```python
from build123d import *

# Parameters (mm, degrees)
F2_R    = 1
F3_SIZE = 1
F4_SIZE = 0.5


with BuildPart() as f1:
    # F0 (on Front) → F1 (revolve)
    with BuildSketch(Plane.XZ):
        Polygon((0, 7.5), (-10.669873, 7.5), (-15, 0), (0, 0), (0, 2), (15, 2), (15, 4), (0, 4), align=None)
    revolve(axis=Axis((-7.5, 0, 0), (1, 0, 0)))

    # F2
    f2_edges = [f1.edges().sort_by_distance(p)[0] for p in [
        (-10.669873, 0, -7.5),
    ]]
    fillet(f2_edges, radius=F2_R)

    # F3
    f3_edges = [f1.edges().sort_by_distance(p)[0] for p in [
        (0, 0, -7.5),
    ]]
    chamfer(f3_edges, length=F3_SIZE)

    # F4
    f4_edges = [f1.edges().sort_by_distance(p)[0] for p in [
        (15, 0, -4),
    ]]
    chamfer(f4_edges, length=F4_SIZE)


solid = f1.part
```
Check sheet for the modelled part. Datum: model origin and axes. Units: mm. A direction names the side the tool comes from. Coordinates: 2 decimals unless noted, no trailing zeros. Order: outer loops, then holes, each group sorted by start corner. A loop starts at its lowest first (then second) coordinate and runs counter-clockwise, first axis right, second up. Notation, with made-up numbers: M 85.25,-25.5 L 144.25,-25.5 A24 ccw 144.25,-14.5 Z; hole C 47,34.5 d11. An arc over 180 degrees is marked long. One line per question, with ' | ' between items. Start each with the question number.
Item 1: Material ranges on line 1 (Y direction, x = 7.5, z = 0); line 2 (Y direction, x = 1.5, z = -0.75), recorded low to high.
Item 2: Gauge pin test, flat ends, axial feed: P1, Ø5, axis at x = 2, z = 5.5, coming from the +Y side; P2, Ø5, axis at x = 8.5, z = 4, coming from the +Y side; P3, Ø4, axis at y = -0.5, z = -4, coming from the -X side. Record the tip position at first contact, or that the pin passes through.
Item 3: Access from +Z, -Z, +X, -X, +Y, -Y to the whole of each face (thin tool, end or side, straight path). Record for faces 1 (the cylindrical face through (-5.61, 2.87, 6.93)), 2 (the flat face through (0, -3, -3)).
Item 4: Mould release check, pull along Z, two halves, no side actions. Record for faces 3 (the cylindrical face through (7.148, 3.905, -0.867)), 4 (the flat face through (15, 2, -2)), 5 (the cylindrical face through (8, 2, 0)), 6 (the flat face through (0, 0, 0)): pulls with the +Z half, pulls with the -Z half, needs draft (parallel to the pull), parting line crosses it, or undercut.
Item 5: Sectioned sample at B-B on x = -5. Record the cut outline in (y, z).
Item 6: Sectioned sample at A-A on x = 12.5. Record the cut outline in (y, z).
Answer below:
1) line 1: y = -4 to -2, 2 to 4 | line 2: y = -3.93 to -1.85, 1.85 to 3.93
2) P1: stops at y = 5.14 | P2: stops at y = 3.71 | P3: stops at x = -13.83
3) face 1: +X, -X | face 2: +X
4) face 3: parting line crosses it | face 4: needs draft | face 5: undercut | face 6: undercut
5) outline: C 0,0 d15
6) outline: C 0,0 d8; hole C 0,0 d4
